Geometry check sheet. Reference: the model listing, model coordinates, mm. A direction names the side the tool comes from. Give positions to 0.01 mm unless a question says otherwise; leave off trailing zeros. Order: outer loops, then holes, each group sorted by start corner. A loop starts at its lowest first (then second) coordinate and runs counter-clockwise, first axis right, second up. Notation, with made-up numbers: (89.5, 16) - (145.5, 16) arc R14 ccw to (145.5, 27) - close; hole circle Ø5 at (15.5, -20.5). An arc over 180 degrees is marked (long way). Put each result on its own line as item: value. Start each with the question number.
```python
from build123d import *

# Parameters (mm, degrees)
F0_W      = 275.59
F0_H      = 416.052
F1_DEPTH  = 406.4
F3_DEPTH  = 406.401
F4_W      = 355.6
F4_H      = 25.4
F5_DEPTH  = 275.591
F6_R      = 31.75
F7_R      = 25.4
F8_R      = 31.75
F10_DEPTH = 3.175


with BuildPart() as f1:
    # F0 (on Front) → F1 (new body)
    with BuildSketch(Plane.XZ):
        with Locations((137.795, 208.026)):
            Rectangle(F0_W, F0_H)
    extrude(amount=-F1_DEPTH)

    # F2 (on face) → F3 (cut, through all)
    with BuildSketch(Plane.XZ):
        Polygon((8.89, 31.75), (8.89, 0), (137.795, 0), (266.7, 0), (266.7, 31.75), (137.795, 31.75), align=None)
    extrude(amount=-F3_DEPTH, mode=Mode.SUBTRACT)

    # F4 (on face) → F5 (cut, through all)
    with BuildSketch(Plane(origin=(0, 0, 0), x_dir=(0, -1, 0), z_dir=(-1, 0, 0))):
        with Locations((-228.6, 403.352)):
            Rectangle(F4_W, F4_H)
        with BuildLine():
            ThreePointArc((-330.2, 31.75), (-326.480256, 22.769744), (-317.5, 19.05))
            Line((-317.5, 19.05), (-101.6, 19.05))
            ThreePointArc((-101.6, 19.05), (-92.619744, 22.769744), (-88.9, 31.75))
            Line((-88.9, 31.75), (-330.2, 31.75))
        make_face()
    extrude(amount=-F5_DEPTH, mode=Mode.SUBTRACT)

    # F6
    f6_edges = [f1.edges().sort_by_distance(p)[0] for p in [
        (4.445, 406.4, 0),
        (271.145, 406.4, 0),
        (271.145, 0, 0),
        (4.445, 0, 0),
    ]]
    fillet(f6_edges, radius=F6_R)

    # F7
    f7_edges = [f1.edges().sort_by_distance(p)[0] for p in [
        (0, 228.6, 390.652),
        (275.59, 228.6, 390.652),
    ]]
    fillet(f7_edges, radius=F7_R)

    # F8
    f8_edges = [f1.edges().sort_by_distance(p)[0] for p in [
        (275.59, 25.4, 416.052),
        (0, 25.4, 416.052),
    ]]
    fillet(f8_edges, radius=F8_R)

    # F9 (on face) → F10 (cut)
    with BuildSketch(Plane.XZ):
        with BuildLine():
            Line((8.89, 384.302), (8.89, 31.75))
            Line((8.89, 31.75), (266.7, 31.75))
            Line((266.7, 31.75), (266.7, 384.302))
            ThreePointArc((266.7, 384.302), (260.004461, 400.466461), (243.84, 407.162))
            Line((243.84, 407.162), (31.75, 407.162))
            ThreePointArc((31.75, 407.162), (15.585539, 400.466461), (8.89, 384.302))
        make_face()
    extrude(amount=-F10_DEPTH, mode=Mode.SUBTRACT)


solid = f1.part
```
Item 1: Release check for a two-part mould opening along Z. For faces 5 (the face through (15.76, 1.57, 400.64)), 6 (the face through (266.54, 25.76, 406.5)), 7 (the face through (271.08, 326.58, 22.87)) record: +Z half, -Z half, draft (parallel to the pull), parting line (faces both ways), or undercut.
Item 2: Cross-section at C-C (y = 352.5). Enter the section's corners in (x, z).
Item 3: Cross-section at B-B (x = 217.5). Enter the section's corners in (y, z) (3 decimals).
Item 4: Cross-section at D-D (x = 259). Enter the section's corners in (y, z) (3 decimals), and give its area (3 significant figures).
Item 5: Cross-section at A-A (y = 172). Enter the section's corners in (x, z), and give its area (3 significant figures).
Item 6: Thickness scan on line 1 along Y through (x, z) = (209, 326) (3 decimals); line 2 along Y through (x, z) = (45, 393) (3 decimals); line 3 along Z through (x, y) = (115.5, 176). Record the ranges inside material, lowest first.
Item 7: Gauge pin test, flat ends, axial feed: pin 1 Ø10 at (x, y) = (6, 166) entering from +Z; pin 2 Ø1.5 at (x, z) = (206, 346.5) entering from -Y (3 decimals); pin 3 Ø3 at (x, y) = (157, 257) entering from -Z. Record the tip position at first contact, or that the pin passes through.
Item 8: Set-up check for faces 1 (the face through (136, 3.175, 222)), 2 (the face through (4.38, 92.72, 22.67)), 3 (the face through (7.24, 226.11, 383.01)), 4 (the face through (136, 231, 390.652)): record each of +Z, -Z, +X, -X, +Y, -Y from which the full face is reachable in a straight line by a thin tool's end or side.
Recorded:
1. face 5: -Z half
1. face 6: +Z half
1. face 7: undercut
2. outline: (0, 0) - (8.89, 0) - (8.89, 31.75) - (266.7, 31.75) - (266.7, 0) - (275.59, 0) - (275.59, 365.25) arc R25.4 ccw to (250.19, 390.65) - (25.4, 390.65) arc R25.4 ccw to (0, 365.25) - close
3. outline: (0, 407.162) - (3.175, 407.162) - (3.175, 31.75) - (406.4, 31.75) - (406.4, 390.652) - (50.8, 390.652) - (50.8, 416.052) - (0, 416.052) - close
4. outline: (0, 401.412) - (3.175, 401.412) - (3.175, 31.75) - (406.4, 31.75) - (406.4, 389.075) - (50.8, 389.075) - (50.8, 412.199) - (0, 412.199) - close
4. area: 145,000 mm^2
5. outline: (0, 0) - (8.89, 0) - (8.89, 19.05) - (0, 19.05) - close; (0, 31.75) - (275.59, 31.75) - (275.59, 365.25) arc R25.4 ccw to (250.19, 390.65) - (25.4, 390.65) arc R25.4 ccw to (0, 365.25) - close; (266.7, 0) - (275.59, 0) - (275.59, 19.05) - (266.7, 19.05) - close
5. area: 99,000 mm^2
6. line 1: y = 3.175 to 406.4
6. line 2: y = 3.175 to 50.8
6. line 3: z = 31.75 to 390.65
7. pin 1: stops at z = 386.18
7. pin 2: stops at y = 3.175
7. pin 3: stops at z = 31.75
8. face 1: -Z, -Y
8. face 2: +X, -X
8. face 3: +Z, -X, +Y
8. face 4: +Z, +X, -X, +Y
